```python
from build123d import *

# Parameters (mm, degrees)
F1_DEPTH = 1.5
F2_W     = 63.5
F2_H     = 0.5
F3_DEPTH = 4
F4_W     = 47.5
F4_H     = 39.9
F4_H_2   = 39.2
F5_DEPTH = 1.501
F6_R     = 8


with BuildPart() as f1:
    # F0 (on Top) → F1 (new body)
    with BuildSketch(Plane.XY):
        Polygon((0, 11.5), (0, 0), (63.5, 0), (63.5, 11.7), (68.1, 10.2), (68.1, 17.8), (63.5, 16.3), (63.5, 29.5), (58.5, 28), (58.5, 36), (63.5, 34.5), (63.5, 64), (68.1, 62.5), (68.1, 70.3), (63.5, 68.8), (63.5, 82), (58.5, 80.5), (58.5, 88.5), (63.5, 87), (63.5, 116.6), (68.1, 115.1), (68.1, 122.9), (63.5, 121.4), (63.5, 134.5), (58.5, 133), (58.5, 141), (63.5, 139.5), (63.5, 151), (0, 151), (0, 139.4), (-4.6, 140.9), (-4.6, 133.1), (0, 134.6), (0, 121.5), (5, 123), (5, 115), (0, 116.5), (0, 86.65), (-4.6, 88.15), (-4.6, 80.35), (0, 81.85), (0, 68.75), (5, 70.25), (5, 62.25), (0, 63.75), (0, 34.3), (-4.6, 35.8), (-4.6, 28.2), (0, 29.7), (0, 16.5), (5, 18), (5, 10), align=None)
    extrude(amount=F1_DEPTH)

    # F2 (on face) → F3 (join)
    with BuildSketch(Plane.XY.offset(1.5)):
        with Locations((31.75, 0.25)):
            Rectangle(F2_W, F2_H)
        with Locations((31.75, 150.75)):
            Rectangle(F2_W, F2_H)
    extrude(amount=F3_DEPTH)

    # F4 (on face) → F5 (cut, through all)
    with BuildSketch(Plane.XY.offset(1.5)):
        with Locations((31.75, 123.05)):
            Rectangle(F4_W, F4_H)
        with Locations((31.75, 75.5)):
            Rectangle(F4_W, F4_H_2)
        with Locations((31.75, 27.95)):
            Rectangle(F4_W, F4_H)
    extrude(amount=-F5_DEPTH, mode=Mode.SUBTRACT)

    # F6
    f6_edges = [f1.edges().sort_by_distance(p)[0] for p in [
        (8, 143, 0.75),
        (8, 95.1, 0.75),
        (8, 47.9, 0.75),
        (8, 103.1, 0.75),
        (8, 55.9, 0.75),
        (8, 8, 0.75),
        (55.5, 8, 0.75),
        (55.5, 55.9, 0.75),
        (55.5, 103.1, 0.75),
        (55.5, 143, 0.75),
        (55.5, 95.1, 0.75),
        (55.5, 47.9, 0.75),
    ]]
    fillet(f6_edges, radius=F6_R)


solid = f1.part
```
Geometry: final body of the model. Coordinates: model frame, mm. A direction names the side the tool comes from. Coordinates: 2 decimals unless noted, no trailing zeros. Order: outer loops, then holes, each group sorted by start corner. A loop starts at its lowest first (then second) coordinate and runs counter-clockwise, first axis right, second up. Notation, with made-up numbers: (80, -31.5) - (104, -31.5) arc R34 cw to (104, 3.5) - close; hole circle Ø8 at (-19, 84). An arc over 180 degrees is marked (long way). Write each question's results on one line, items separated by ' | '.
1) Section B-B, the plane x = 22. Return loops of the section in (y, z).
Results list:
outline: (0, 0) - (8, 0) - (8, 1.5) - (0.5, 1.5) - (0.5, 5.5) - (0, 5.5) - close; (47.9, 0) - (55.9, 0) - (55.9, 1.5) - (47.9, 1.5) - close; (95.1, 0) - (103.1, 0) - (103.1, 1.5) - (95.1, 1.5) - close; (143, 0) - (151, 0) - (151, 5.5) - (150.5, 5.5) - (150.5, 1.5) - (143, 1.5) - close
2) Line query: line 1 (Y direction, x = 17, z = 0.9); line 2 (Y direction, x = 16.5, z = 4.3); line 3 (X direction, y = 20.5, z = 0.55). Output: solid intervals per line, ascending. Write a range as from..to.
Results list:
line 1: 0..8, 47.9..55.9, 95.1..103.1, 143..151 | line 2: 0..0.5, 150.5..151 | line 3: 0..8, 55.5..63.5
3) Section D-D, the plane x = 52. Return loops of the section in (y, z).
Results list:
outline: (0, 0) - (9.39, 0) - (9.39, 1.5) - (0.5, 1.5) - (0.5, 5.5) - (0, 5.5) - close; (46.51, 0) - (57.29, 0) - (57.29, 1.5) - (46.51, 1.5) - close; (93.71, 0) - (104.49, 0) - (104.49, 1.5) - (93.71, 1.5) - close; (141.61, 0) - (151, 0) - (151, 5.5) - (150.5, 5.5) - (150.5, 1.5) - (141.61, 1.5) - close
4) Section A-A, the plane y = 113. Return loops of the section in (x, z).
Results list:
outline: (0, 0) - (8, 0) - (8, 1.5) - (0, 1.5) - close; (55.5, 0) - (63.5, 0) - (63.5, 1.5) - (55.5, 1.5) - close
5) Pull-direction query (Y, two-part tool) for faces 1 (the flat face through (32, 151, 3)), 2 (the flat face through (31, 0.5, 3)), 3 (the flat face through (0, 146, 1)); classes: pulls with the +Y half, pulls with the -Y half, needs draft (parallel to the pull), parting line crosses it, or undercut.
Results list:
face 1: pulls with the +Y half | face 2: undercut | face 3: needs draft
6) Section C-C, the plane z = 3.1. Return loops of the section in (x, y), plus the area to 3 significant figures.
Results list:
outline: (0, 0) - (63.5, 0) - (63.5, 0.5) - (0, 0.5) - close; (0, 150.5) - (63.5, 150.5) - (63.5, 151) - (0, 151) - close | area: 63.5 mm^2
7) Set-up query: faces 4 (the flat face through (26, 98, 1.5)), 5 (the flat face through (63.5, 146, 1)), 6 (the cylindrical face through (53.094, 10.281, 0.74)), 7 (the flat face through (0, 5, 1)). Return all of +Z, -Z, +X, -X, +Y, -Y with unobstructed straight access to the full face (end or side cutting, diameter ignored); none if empty.
Results list:
face 4: +Z, +X, -X | face 5: +Z, -Z, +X, +Y | face 6: +Z, -Z | face 7: +Z, -Z, -X, -Y
8) Pin query (flat end, axial travel): pin 1 (1.6 mm diameter, centred on y = 137.5, z = 1, fed in from +X); pin 2 (0.8 mm diameter, centred on y = 50, z = 1, fed in from -X); pin 3 (1.6 mm diameter, centred on y = 120.5, z = 1, fed in from -X); pin 4 (1.2 mm diameter, centred on x = 29, z = 1, fed in from -Y). Return the tip coordinate at first contact, or that it passes through.
Results list:
pin 1: x = 58.5 | pin 2: x = 0 | pin 3: x = 5 | pin 4: y = 0
